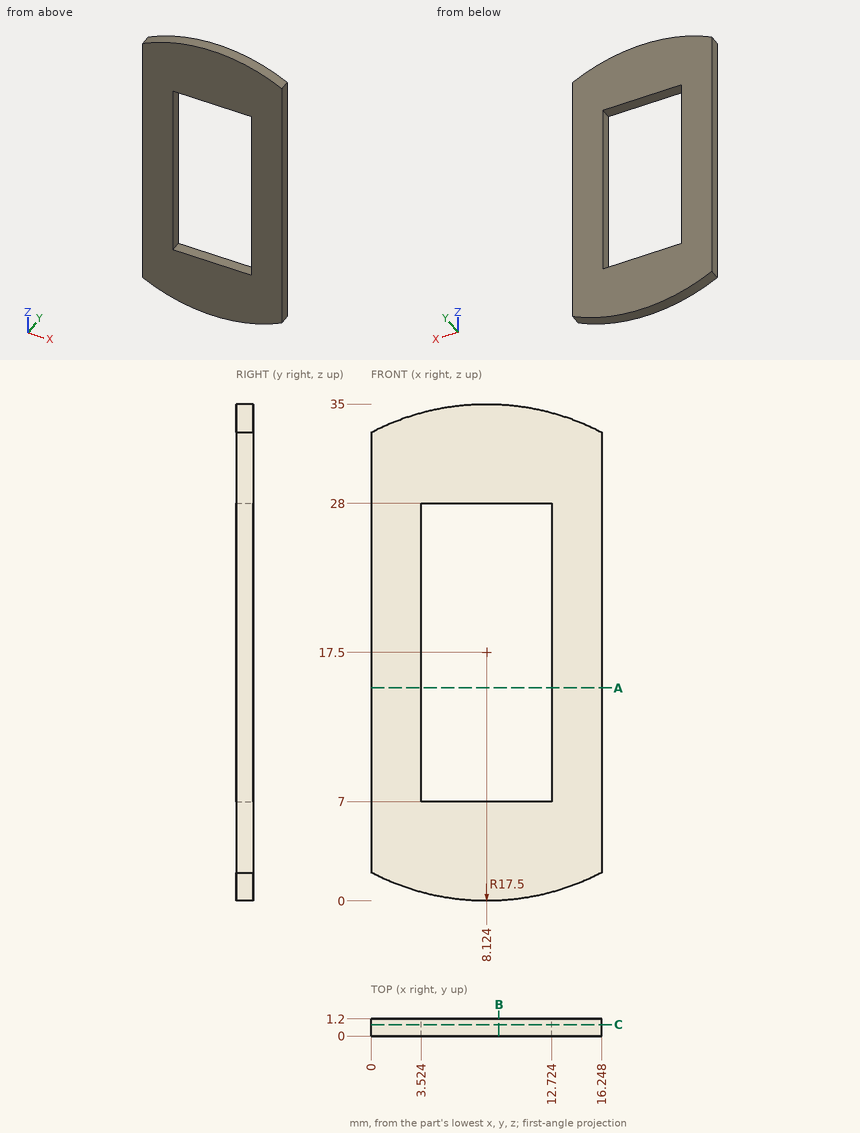
Source: three-view drawing plus pictorial views. Frame: mm from the lowest corner of the part. Coordinates: 2 decimals unless noted, no trailing zeros. Write each loop counter-clockwise with the first axis right and the second up, starting at its lowest first coordinate (ties: lowest second). Pieces come first, ordered by that corner, then holes. Notation, with made-up numbers: (83, 88.25) -> (115, 88.25) arc R19 cw to (115, 95.25) -> close; hole circle Ø11 at (89, 73). An arc over 180 degrees is marked (long way). Answer as a JSON object with one key per item and string values.
1. Section C-C on y = 0.8. Return the cut outline in (x, z), then the cut area to 3 significant figures.
Result set:
{"outline": "(0, 2) arc R17.5 ccw to (16.25, 2) -> (16.25, 33) arc R17.5 ccw to (0, 33) -> close; hole (3.52, 7) -> (12.72, 7) -> (12.72, 28) -> (3.52, 28) -> close", "area": "354 mm2"}
2. Section A-A on z = 15. Return the cut outline in (x, y).
Result set:
{"outline": "(0, 0) -> (3.52, 0) -> (3.52, 1.2) -> (0, 1.2) -> close; (12.72, 0) -> (16.25, 0) -> (16.25, 1.2) -> (12.72, 1.2) -> close"}
3. Section B-B on x = 9. Return the cut outline in (y, z).
Result set:
{"outline": "(0, 0.02) -> (1.2, 0.02) -> (1.2, 7) -> (0, 7) -> close; (0, 28) -> (1.2, 28) -> (1.2, 34.98) -> (0, 34.98) -> close"}
4. Material intervals for line 1 (Z direction, x = 8.5, y = 0.65); line 2 (X direction, y = 0.6, z = 11); line 3 (Z direction, x = 5.5, y = 0.8), sorted ascending. Write a range as from..to.
Result set:
{"line 1": "z = 0..7, 28..35", "line 2": "x = 0..3.52, 12.72..16.25", "line 3": "z = 0.2..7, 28..34.8"}
